Geometry: final body of the model. Coordinates: model frame, mm. Round coordinates to 2 decimals unless told otherwise and drop trailing zeros. Loops run counter-clockwise (first coordinate to the right, second up) from the corner with the lowest first, then second, coordinate; pieces in that order, holes last. Notation, with made-up numbers: (-40, 3) - (-10, 3) arc R14 ccw to (-10, 28) - close; hole circle Ø1 at (-31.5, -10). An arc over 180 degrees is marked (long way). Answer as a JSON object with one key per item and string values. Group by question number.
Item 1: First-contact query: pin 1 (1 mm diameter, centred on y = 2, z = 1.5, fed in from +X). Flat tip, straight axial feed; report the tip coordinate or a pass-through.
Item 2: Line query: line 1 (Y direction, x = 0, z = 2); line 2 (X direction, y = 10.5, z = 2.15); line 3 (X direction, y = -7, z = 1). Output: solid intervals per line, ascending.
Item 3: Section A-A (x = 0). Return the cut outline in (y, z).
Item 4: Section B-B (z = 2.5). Return the cut outline in (x, y) (3 decimals).
```python
from build123d import *

# Parameters (mm, degrees)
F0_R     = 19.5
F1_DEPTH = 3.3
F2_R     = 0.254
F3_R     = 0.635
F4_DEPTH = 4


with BuildPart() as f1:
    # F0 (on Top) → F1 (new body)
    with BuildSketch(Plane.XY):
        Circle(F0_R)
    extrude(amount=F1_DEPTH)

    # F2
    f2_edges = [f1.edges().sort_by_distance(p)[0] for p in [
        (-19.5, 0, 3.3),
        (-19.5, 0, 0),
    ]]
    fillet(f2_edges, radius=F2_R)

    # F3 (on face) → F4 (cut)
    with BuildSketch(Plane(origin=(0, 0, 0), x_dir=(1, 0, 0), z_dir=(0, 0, -1))):
        with Locations((0, 15.682086)):
            Circle(F3_R)
    extrude(amount=-F4_DEPTH, mode=Mode.SUBTRACT)


solid = f1.part
```
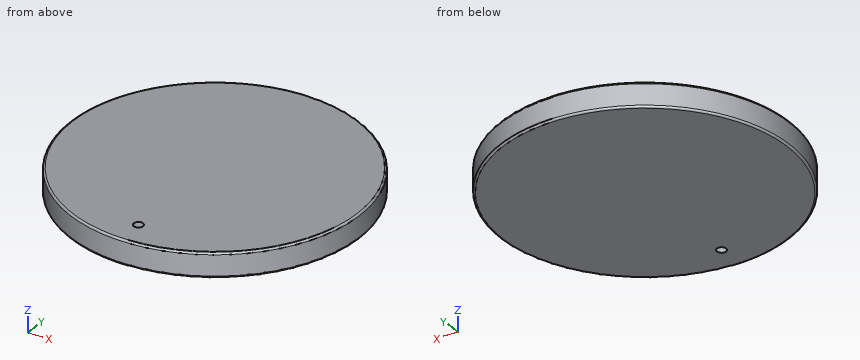
Values:
{
 "1": {"pin 1": "stops at x = 19.44"},
 "2": {"line 1": "y = -19.5 to -16.32, -15.05 to 19.5", "line 2": "x = -16.43 to 16.43", "line 3": "x = -18.2 to 18.2"},
 "3": {"outline": "(-19.5, 0.25) arc R0.25 ccw to (-19.25, 0) - (-16.32, 0) - (-16.32, 3.3) - (-19.25, 3.3) arc R0.25 ccw to (-19.5, 3.05) - close; (-15.05, 0) - (19.25, 0) arc R0.25 ccw to (19.5, 0.25) - (19.5, 3.05) arc R0.25 ccw to (19.25, 3.3) - (-15.05, 3.3) - close"},
 "4": {"outline": "circle Ø39 at (0, 0); hole circle Ø1.27 at (0, -15.682)"}
}
